from build123d import *

# Parameters (mm, degrees)
SKETCH1_W           = 12.2
SKETCH1_H           = 12.2
BOSS_EXTRUDE1_DEPTH = 120
SKETCH2_OUTSIDE_W   = 38.446
SKETCH2_OUTSIDE_H   = 38.446
SKETCH2_OUTSIDE_R   = 6.95
CUT_EXTRUDE1_DEPTH  = 121.309683733
SKETCH3_OUTSIDE_W   = 41.946
SKETCH3_OUTSIDE_H   = 41.946
SKETCH3_OUTSIDE_R   = 5.3
CUT_EXTRUDE2_DEPTH  = 20
CUT_EXTRUDE2_DRAFT  = -5
CUT_EXTRUDE3_START  = -60
SKETCH4_OUTSIDE_W   = 38.446
SKETCH4_OUTSIDE_H   = 38.446
SKETCH4_OUTSIDE_R   = 6.1
CUT_EXTRUDE3_DEPTH  = 50
SKETCH5_OUTSIDE_W   = 40.11
SKETCH5_OUTSIDE_H   = 40.11
SKETCH5_OUTSIDE_R   = 6.1
CUT_EXTRUDE4_DEPTH  = 9.5
CUT_EXTRUDE4_DRAFT  = -5
BOSS_EXTRUDE2_DEPTH = 3.5
SKETCH6_OUTSIDE_W   = 40.78
SKETCH6_OUTSIDE_H   = 40.78
SKETCH6_OUTSIDE_R   = 6.1
CUT_EXTRUDE6_DEPTH  = 9.5
CUT_EXTRUDE6_DRAFT  = -7
SKETCH8_OUTSIDE_W   = 68.768
SKETCH8_OUTSIDE_H   = 68.768
SKETCH8_OUTSIDE_R   = 4.5
CUT_EXTRUDE7_DEPTH  = 3.5
CUT_EXTRUDE7_DRAFT  = -77
BOSS_EXTRUDE3_DEPTH = 16


with BuildPart() as part:
    # Sketch1 → Boss-Extrude1 (new body)
    with BuildSketch(Plane.XY):
        Rectangle(SKETCH1_W, SKETCH1_H)
    extrude(amount=BOSS_EXTRUDE1_DEPTH)

    # Sketch2 outside → Cut-Extrude1 (cut, through all)
    with BuildSketch(Plane.XY.offset(120)):
        Rectangle(SKETCH2_OUTSIDE_W, SKETCH2_OUTSIDE_H)
        Circle(SKETCH2_OUTSIDE_R, mode=Mode.SUBTRACT)
    extrude(amount=-CUT_EXTRUDE1_DEPTH, mode=Mode.SUBTRACT)


with BuildPart() as cut_extrude2_tool:
    # Sketch3 outside → Cut-Extrude2 (with draft: the straight prism first)
    with BuildSketch(Plane.XY.offset(120)):
        Rectangle(SKETCH3_OUTSIDE_W, SKETCH3_OUTSIDE_H)
        Circle(SKETCH3_OUTSIDE_R, mode=Mode.SUBTRACT)
    extrude(amount=-CUT_EXTRUDE2_DEPTH)
    # Cut-Extrude2: the draft: its side faces are tilted about the plane it starts from
    cut_extrude2_sides = [cut_extrude2_tool.faces().sort_by_distance(p)[0] for p in [
        (0, -20.973, 110),
        (20.973, 0, 110),
        (0, 20.973, 110),
        (-20.973, 0, 110),
        (-5.3, 0, 110),
    ]]
    draft(cut_extrude2_sides, Plane.XY.offset(120), CUT_EXTRUDE2_DRAFT)


with BuildPart() as part_1:
    add(part.part)

    # Cut-Extrude2: cut by cut_extrude2_tool
    add(cut_extrude2_tool.part, mode=Mode.SUBTRACT)

    # Sketch4 outside → Cut-Extrude3 (cut)
    with BuildSketch(Plane.XY.offset(120).offset(CUT_EXTRUDE3_START)):
        Rectangle(SKETCH4_OUTSIDE_W, SKETCH4_OUTSIDE_H)
        Circle(SKETCH4_OUTSIDE_R, mode=Mode.SUBTRACT)
    extrude(amount=-CUT_EXTRUDE3_DEPTH, mode=Mode.SUBTRACT)


with BuildPart() as cut_extrude4_tool:
    # Sketch5 outside → Cut-Extrude4 (with draft: the straight prism first)
    with BuildSketch(Plane(origin=(0, 0, 60), x_dir=(-1, 0, 0), z_dir=(0, 0, -1))):
        Rectangle(SKETCH5_OUTSIDE_W, SKETCH5_OUTSIDE_H)
        with Locations(Location((0, 0, 0), (0, 0, 180))):
            Circle(SKETCH5_OUTSIDE_R, mode=Mode.SUBTRACT)
    extrude(amount=-CUT_EXTRUDE4_DEPTH)
    # Cut-Extrude4: the draft: its side faces are tilted about the plane it starts from
    cut_extrude4_sides = [cut_extrude4_tool.faces().sort_by_distance(p)[0] for p in [
        (0, -20.055, 64.75),
        (-20.055, 0, 64.75),
        (0, 20.055, 64.75),
        (20.055, 0, 64.75),
        (-6.1, 0, 64.75),
    ]]
    draft(cut_extrude4_sides, Plane(origin=(0, 0, 60), x_dir=(-1, 0, 0), z_dir=(0, 0, -1)), CUT_EXTRUDE4_DRAFT)


with BuildPart() as part_2:
    add(part_1.part)

    # Cut-Extrude4: cut by cut_extrude4_tool
    add(cut_extrude4_tool.part, mode=Mode.SUBTRACT)

    # Sketch7 → Boss-Extrude2 (add)
    with BuildSketch(Plane(origin=(0, 0, 0), x_dir=(-1, 0, 0), z_dir=(0, 0, -1))):
        with BuildLine():
            Line((3.433656943, -6.1), (-3.433656943, -6.1))
            ThreePointArc((-3.433656943, -6.1), (-4.949747468, -4.949747468), (-6.1, -3.433656943))
            Line((-6.1, -3.433656943), (-6.1, 3.433656943))
            ThreePointArc((-6.1, 3.433656943), (-4.949747468, 4.949747468), (-3.433656943, 6.1))
            Line((-3.433656943, 6.1), (3.433656943, 6.1))
            ThreePointArc((3.433656943, 6.1), (4.949747468, 4.949747468), (6.1, 3.433656943))
            Line((6.1, 3.433656943), (6.1, -3.433656943))
            ThreePointArc((6.1, -3.433656943), (4.949747468, -4.949747468), (3.433656943, -6.1))
        make_face()
    extrude(amount=-BOSS_EXTRUDE2_DEPTH)


with BuildPart() as cut_extrude6_tool:
    # Sketch6 outside → Cut-Extrude6 (with draft: the straight prism first)
    with BuildSketch(Plane.XY.offset(10)):
        Rectangle(SKETCH6_OUTSIDE_W, SKETCH6_OUTSIDE_H)
        Circle(SKETCH6_OUTSIDE_R, mode=Mode.SUBTRACT)
    extrude(amount=-CUT_EXTRUDE6_DEPTH)
    # Cut-Extrude6: the draft: its side faces are tilted about the plane it starts from
    cut_extrude6_sides = [cut_extrude6_tool.faces().sort_by_distance(p)[0] for p in [
        (0, -20.39, 5.25),
        (20.39, 0, 5.25),
        (0, 20.39, 5.25),
        (-20.39, 0, 5.25),
        (-6.1, 0, 5.25),
    ]]
    draft(cut_extrude6_sides, Plane.XY.offset(10), CUT_EXTRUDE6_DRAFT)


with BuildPart() as part_3:
    add(part_2.part)

    # Cut-Extrude6: cut by cut_extrude6_tool
    add(cut_extrude6_tool.part, mode=Mode.SUBTRACT)


with BuildPart() as cut_extrude7_tool:
    # Sketch8 outside → Cut-Extrude7 (with draft: the straight prism first)
    with BuildSketch(Plane(origin=(0, 0, 0), x_dir=(-1, 0, 0), z_dir=(0, 0, -1))):
        Rectangle(SKETCH8_OUTSIDE_W, SKETCH8_OUTSIDE_H)
        Circle(SKETCH8_OUTSIDE_R, mode=Mode.SUBTRACT)
    extrude(amount=-CUT_EXTRUDE7_DEPTH)
    # Cut-Extrude7: the draft: its side faces are tilted about the plane it starts from
    cut_extrude7_sides = [cut_extrude7_tool.faces().sort_by_distance(p)[0] for p in [
        (0, -34.384, 1.75),
        (-34.384, 0, 1.75),
        (0, 34.384, 1.75),
        (34.384, 0, 1.75),
        (4.5, 0, 1.75),
    ]]
    draft(cut_extrude7_sides, Plane(origin=(0, 0, 0), x_dir=(-1, 0, 0), z_dir=(0, 0, -1)), CUT_EXTRUDE7_DRAFT)


with BuildPart() as part_4:
    add(part_3.part)

    # Cut-Extrude7: cut by cut_extrude7_tool
    add(cut_extrude7_tool.part, mode=Mode.SUBTRACT)

    # Sketch9 → Boss-Extrude3 (add)
    with BuildSketch(Plane.XY.offset(120)):
        Polygon((1.732050808, 3), (-1.732050808, 3), (-3.464101615, 0), (-1.732050808, -3), (1.732050808, -3), (3.464101615, 0), align=None)
    extrude(amount=BOSS_EXTRUDE3_DEPTH)

    # Sketch10 → Cut-Revolve1 (revolve, cut)
    with BuildSketch(Plane(origin=(0, 0, 0), x_dir=(1, 0, 0), z_dir=(0, 1, 0))):
        with BuildLine():
            Line((3, -136), (3, -126))
            ThreePointArc((3, -126), (3.1186767, -125.214921929), (3.464101615, -124.5))
            Line((3.464101615, -124.5), (3.464101615, -136))
            Line((3.464101615, -136), (3, -136))
        make_face()
    revolve(axis=Axis((0, 0, 120), (0, 0, -1)), mode=Mode.SUBTRACT)


solid = part_4.part
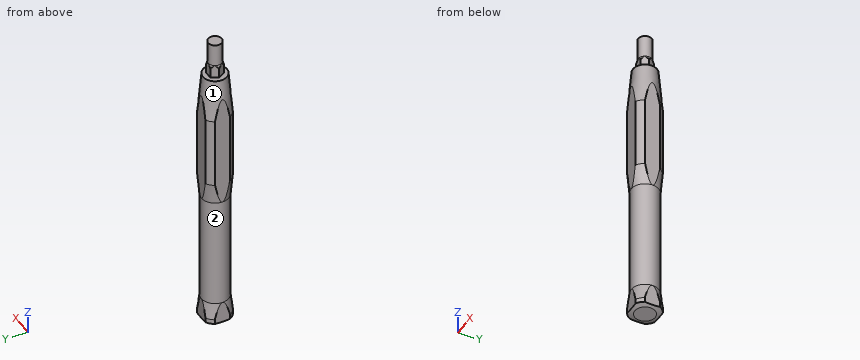
CAD build for the part. Positions are in the model's coordinates, mm. Face numbers are marked on the shaded views. Coordinates: 2 decimals unless noted, no trailing zeros. Order: outer loops, then holes, each group sorted by start corner. A loop starts at its lowest first (then second) coordinate and runs counter-clockwise, first axis right, second up. Notation, with made-up numbers: (47.25, -7.5) -> (76.25, -7.5) arc R24 ccw to (76.25, 6.5) -> close; hole circle Ø11 at (24.5, 78.5). An arc over 180 degrees is marked (long way). Answer in a Markdown table with one row per item.
1) Band-saw the part on B-B (z = 48). List the corners of the cut face in (x, y).
Check values:
| item | result |
|---|---|
| outline | circle Ø12.2 at (0, 0) |
2) Drill centre lines: line 1 (Z direction, x = -1.75, y = 3.5); line 2 (Y direction, x = 0.5, z = 28.5); line 3 (Y direction, x = -5.5, z = 41). Where is each one in solid material? Low to high.
Check values:
| item | result |
|---|---|
| line 1 | 0 to 120 |
| line 2 | -6.08 to 6.08 |
| line 3 | -2.64 to 2.64 |
3) Flat gauge pins, fed straight in: P1, Ø0.8, axis at x = -5, y = 5, coming from the -Z side; P2, Ø0.8, axis at x = 4, y = -4.5, coming from the -Z side; P3, Ø6, axis at x = -4.5, z = 59, coming from the -Y side. Where does each tip first touch, or does it go through?
Check values:
| item | result |
|---|---|
| P1 | z = 0.5 |
| P2 | z = 0.26 |
| P3 | y = -5.91 |
4) Mould opens along Z. For the marked faces 1 and 2 say: pulls with the +Z half, pulls with the -Z half, needs draft (parallel to the pull), parting line crosses it, or undercut.
Check values:
| item | result |
|---|---|
| face 1 | pulls with the +Z half |
| face 2 | undercut |
5) Band-saw the part on C-C (z = 107). List the corners of the cut face in (x, y).
Check values:
| item | result |
|---|---|
| outline | (-6.1, -2.06) arc R6.44 ccw to (-2.06, -6.1) -> (2.06, -6.1) arc R6.44 ccw to (6.1, -2.06) -> (6.1, 2.06) arc R6.44 ccw to (2.06, 6.1) -> (-2.06, 6.1) arc R6.44 ccw to (-6.1, 2.06) -> close |
6) Band-saw the part on A-A (z = 74). List the corners of the cut face in (x, y).
Check values:
| item | result |
|---|---|
| outline | (-6.1, -3.33) arc R6.95 ccw to (-3.33, -6.1) -> (3.33, -6.1) arc R6.95 ccw to (6.1, -3.33) -> (6.1, 3.33) arc R6.95 ccw to (3.33, 6.1) -> (-3.33, 6.1) arc R6.95 ccw to (-6.1, 3.33) -> close |
